from build123d import *

# Parameters (mm, degrees)
ESQUISSE1_W        = 2
ESQUISSE1_H        = 30
BOSS_EXTRU_1_DEPTH = 2.8


with BuildPart() as part:
    # Esquisse1 → Base-Révolution (revolve)
    with BuildSketch(Plane(origin=(0, 0, 0), x_dir=(1, 0, 0), z_dir=(0, 1, 0))):
        with Locations((1, -15)):
            Rectangle(ESQUISSE1_W, ESQUISSE1_H)
    revolve(axis=Axis((0, 0, 0), (0, 0, 1)))

    # Chanfrein1: read off the stored shape, not the designer's step
    # Chanfrein1 outline → Chanfrein1 (revolve, cut)
    with BuildSketch(Plane.XZ):
        Polygon((2, 30), (1.6, 30), (2, 29.6), align=None)
    revolve(axis=Axis((0, 0, 0), (0, 0, 1)), mode=Mode.SUBTRACT)

    # Esquisse6 → Boss.-Extru.1 (add)
    with BuildSketch(Plane.XY):
        Polygon((3.5, -2.020725942), (3.5, 2.020725942), (0, 4.041451884), (-3.5, 2.020725942), (-3.5, -2.020725942), (0, -4.041451884), align=None)
    extrude(amount=-BOSS_EXTRU_1_DEPTH)

    # Esquisse7 → Enlèvement de matière-Révolution1 (revolve, cut)
    with BuildSketch(Plane(origin=(0, 0, 0), x_dir=(1, 0, 0), z_dir=(0, 1, 0))):
        Polygon((-3.5, 2.8), (-8.349742261, 2.8), (-8.349742261, 0), align=None)
    revolve(axis=Axis((0, 0, -6.239446496), (0, 0, 1)), mode=Mode.SUBTRACT)


solid = part.part
Part model, mm, in its own coordinate system. A direction names the side the tool comes from. Coordinates: 2 decimals unless noted, no trailing zeros. Write each loop counter-clockwise with the first axis right and the second up, starting at its lowest first coordinate (ties: lowest second). Pieces come first, ordered by that corner, then holes. Notation, with made-up numbers: (-19.75, 36.5) - (0.25, 36.5) arc R6 ccw to (0.25, 41.5) - close; hole circle Ø1 at (45.5, 71). An arc over 180 degrees is marked (long way). Put each result on its own line as item: value.
1. Flat gauge pins, fed straight in: pin 1 Ø1.5 at (x, z) = (-0.5, 3) entering from +Y; pin 2 Ø3 at (y, z) = (0, 20) entering from -X; pin 3 Ø2 at (y, z) = (-1, 12.5) entering from +X. Where does each tip first touch, or does it go through?
Final values:
pin 1: stops at y = 2
pin 2: stops at x = -2
pin 3: stops at x = 2
2. 3-axis set-ups, long thin cutter, end or side, ignore diameter. For faces 1 (the flat face through (-2, -2, 0)), 2 (the flat face through (-3.5, 0, -1)): which of +Z, -Z, +X, -X, +Y, -Y reach the whole face in a straight line?
Final values:
face 1: +Z
face 2: +Z, -Z, -X, +Y, -Y
3. Band-saw the part on A-A (z = 19). Write the cut outline in (x, y), then the cut area to 3 significant figures.
Final values:
outline: circle Ø4 at (0, 0)
area: 12.6 mm²
4. Probe line 1 along Z through (x, y) = (2.5, -0.75); line 2 along Z through (x, y) = (1, -1.5); line 3 along Y through (x, z) = (0.5, 1.5). List the from-to ranges inside material, lowest first. Write a range as [from, to].
Final values:
line 1: z = [-2.8, 0]
line 2: z = [-2.8, 29.8]
line 3: y = [-1.94, 1.94]
